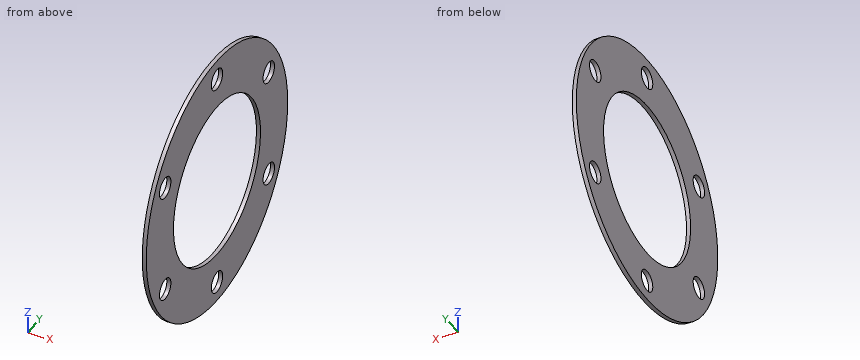
Autodesk Inventor part; units mm, degrees
ref_plane "YZ Plane" through (0, 0, 0) normal (1, 0, 0) x (0, 1, 0)
ref_plane "XZ Plane" through (0, 0, 0) normal (0, 1, 0) x (-1, 0, 0)
ref_plane "XY Plane" through (0, 0, 0) normal (0, 0, 1) x (1, 0, 0)
sketch "Sketch1" plane through (0, 0, 0) normal (1, 0, 0) x (0, 1, 0)
  circle A0 centre (0, 0) radius 65
  dimension "d0" = 130
extrude "Extrusion1" add sketch "Sketch1" along normal blind 2
sketch "Sketch2" plane through (0, 0, 0) normal (-1, 0, 0) x (0, 0, 1)
  circle A0 centre (0, 0) radius 55
  circle A1 centre (-55, 0) radius 5.25
  dimension "d3" = 110
  dimension "d4" = 10.5
hole "Hole1" at (0, 0, -55) direction (1, 0, 0) diameter 10.5 end through all
pattern_circular "Circular Pattern1" count 6 over 360 about axis through (0, 0, 0) along (1, 0, 0) of "Hole1"
sketch "Sketch3" plane through (2, 0, 0) normal (1, 0, 0) x (0, 0, -1)
  circle A0 centre (0, 0) radius 40
  dimension "d15" = 80
extrude "Extrusion2" cut sketch "Sketch3" against normal blind 10
properties part number "08_Dem_dieu_chinh"
Input: part model. Units: mm. Frame: model coordinates. Coordinates: 2 decimals unless noted, no trailing zeros. Order: outer loops, then holes, each group sorted by start corner. A loop starts at its lowest first (then second) coordinate and runs counter-clockwise, first axis right, second up. Notation, with made-up numbers: (-4.75, -26) - (45.25, -26) arc R21 cw to (45.25, -2) - close; hole circle Ø2 at (9, -18.75). An arc over 180 degrees is marked (long way). Put each result on its own line as item: value.
1. Cut plane A-A on y = 0. Return the cut outline in (x, z), then the cut area to 3 significant figures.
Report:
outline: (0, -65) - (2, -65) - (2, -60.25) - (0, -60.25) - close; (0, -49.75) - (2, -49.75) - (2, -40) - (0, -40) - close; (0, 40) - (2, 40) - (2, 49.75) - (0, 49.75) - close; (0, 60.25) - (2, 60.25) - (2, 65) - (0, 65) - close
area: 58.0 mm2
2. Line query: line 1 along Y through (x, z) = (0.75, -27.5); line 2 along Z through (x, y) = (0.15, 48); line 3 along Y through (x, z) = (1.85, 20.5). Output: solid intervals per line, ascending.
Report:
line 1: y = -58.9 to -52.88, -42.38 to -29.05, 29.05 to 42.38, 52.88 to 58.9
line 2: z = -43.83 to -32.74, -22.26 to 22.26, 32.74 to 43.83
line 3: y = -61.68 to -34.35, 34.35 to 61.68
3. Cut plane C-C on y = 26. Return the cut outline in (x, z).
Report:
outline: (0, -59.57) - (2, -59.57) - (2, -30.4) - (0, -30.4) - close; (0, 30.4) - (2, 30.4) - (2, 59.57) - (0, 59.57) - close
4. Cut plane B-B on z = 27.5. Return the cut outline in (x, y).
Report:
outline: (0, -58.9) - (2, -58.9) - (2, -52.88) - (0, -52.88) - close; (0, -42.38) - (2, -42.38) - (2, -29.05) - (0, -29.05) - close; (0, 29.05) - (2, 29.05) - (2, 42.38) - (0, 42.38) - close; (0, 52.88) - (2, 52.88) - (2, 58.9) - (0, 58.9) - close
5. Cut plane D-D on z = 55. Return the cut outline in (x, y), then the cut area to 3 significant figures.
Report:
outline: (0, -34.64) - (2, -34.64) - (2, -5.25) - (0, -5.25) - close; (0, 5.25) - (2, 5.25) - (2, 34.64) - (0, 34.64) - close
area: 118 mm2
6. Contact query for flat-ended pins moving along their axis: pin 1 Ø9.5 at (y, z) = (0, -55) entering from -X; pin 2 Ø17 at (y, z) = (-47.63, 27.5) entering from +X. Output: stop coordinate, or through.
Report:
pin 1: passes through
pin 2: stops at x = 2
